Work out the finished part from the listing and answer in its coordinate system (mm). A direction names the side the tool comes from. Round coordinates to 2 decimals unless told otherwise and drop trailing zeros. Order: outer loops, then holes, each group sorted by start corner. A loop starts at its lowest first (then second) coordinate and runs counter-clockwise, first axis right, second up. Notation, with made-up numbers: (25, -33.5) -> (76, -33.5) arc R26 ccw to (76, -7.5) -> close; hole circle Ø2 at (56.25, -8). An arc over 180 degrees is marked (long way). Use a Markdown table: item, result. Add a question column.
Item 1: A cutting plane is placed at C-C, the plane z = 3.4. Determine the outline of the cut face in (x, y), plus the area to 3 significant figures.
Item 2: A cutting plane is placed at B-B, the plane x = 2.5. Determine the outline of the cut face in (y, z), plus the area to 3 significant figures.
Item 3: For a pull along X with two mould halves and no side action, classify faces 4 (the cylindrical face through (-19, -25.44, 1.01)), 5 (the flat face through (30, 1, 0)), 6 (the flat face through (70, -1, 2)) as +X half, -X half, draft (parallel to the pull), parting line (faces both ways), or undercut.
Item 4: A tool of negligible diameter and unlimited length cuts with its end or side. For faces 1 (the flat face through (-70, -1, 2)), 2 (the cylindrical face through (18.94, -25.5, 1.01)), 3 (the flat face through (-27, 1, 2)), from which of +Z, -Z, +X, -X, +Y, -Y can it reach the whole face along a straight path? Write none if from no direction.
Item 5: Find the intervals of material crossed by L1, parallel to Y at x = -34.5, z = 2.9; L2, parallel to X at y = 10, z = 0.9; L3, parallel to X at y = -17, z = 2.35, in increasing order. Write a range as [from, to].
Item 6: A cutting plane is placed at A-A, the plane y = -32. Determine the outline of the cut face in (x, z), plus the area to 3 significant figures.
Item 7: A cutting plane is placed at D-D, the plane x = -27.5. Determine the outline of the cut face in (y, z).
from build123d import *

# Parameters (mm, degrees)
SKETCH_1_W          = 140
SKETCH_1_H          = 160
EXTRUDE_1_DEPTH     = 2
SKETCH_2_W          = 140
SKETCH_2_H          = 160
SKETCH_2_W_2        = 80
SKETCH_2_H_2        = 100
EXTRUDE_2_DEPTH     = 2
CUT_EXTRUDE_1_DEPTH = 2


with BuildPart() as part:
    # 草图1 → 凸台-拉伸1 (new body)
    with BuildSketch(Plane.XY):
        Rectangle(SKETCH_1_W, SKETCH_1_H)
    extrude(amount=EXTRUDE_1_DEPTH)

    # 草图2 → 凸台-拉伸2 (add)
    with BuildSketch(Plane.XY.offset(2)):
        Rectangle(SKETCH_2_W, SKETCH_2_H)
        Rectangle(SKETCH_2_W_2, SKETCH_2_H_2, mode=Mode.SUBTRACT)
    extrude(amount=EXTRUDE_2_DEPTH)

    # 草图4 → 切除-拉伸1 (cut)
    with BuildSketch(Plane.XY.offset(2)):
        with BuildLine():
            Line((-10.8, -34.2), (-6.8, -34.2))
            Line((-6.8, -34.2), (6.8, -34.2))
            Line((6.8, -34.2), (10.8, -34.2))
            Line((10.8, -34.2), (11.2, -34.2))
            Line((11.2, -34.2), (15.2, -34.2))
            Line((15.2, -34.2), (15.2, -26.7))
            Line((15.2, -26.7), (16, -26.7))
            ThreePointArc((16, -26.7), (18.969848481, -25.469848481), (20.2, -22.5))
            Line((20.2, -22.5), (20.2, 29.5))
            ThreePointArc((20.2, 29.5), (18.969848481, 32.469848481), (16, 33.7))
            Line((16, 33.7), (-16, 33.7))
            ThreePointArc((-16, 33.7), (-18.969848481, 32.469848481), (-20.2, 29.5))
            Line((-20.2, 29.5), (-20.2, -22.5))
            ThreePointArc((-20.2, -22.5), (-18.969848481, -25.469848481), (-16, -26.7))
            Line((-16, -26.7), (-15.2, -26.7))
            Line((-15.2, -26.7), (-15.2, -34.2))
            Line((-15.2, -34.2), (-11.2, -34.2))
            Line((-11.2, -34.2), (-10.8, -34.2))
        make_face()
    extrude(amount=-CUT_EXTRUDE_1_DEPTH, mode=Mode.SUBTRACT)


solid = part.part
Reported:
| question | item | result |
|---|---|---|
| 1 | outline | (-70, -80) -> (70, -80) -> (70, 80) -> (-70, 80) -> close; hole (-40, -50) -> (40, -50) -> (40, 50) -> (-40, 50) -> close |
| 1 | area | 14,400 mm² |
| 2 | outline | (-80, 0) -> (-34.2, 0) -> (-34.2, 2) -> (-50, 2) -> (-50, 4) -> (-80, 4) -> close; (33.7, 0) -> (80, 0) -> (80, 4) -> (50, 4) -> (50, 2) -> (33.7, 2) -> close |
| 2 | area | 304 mm² |
| 3 | face 4 | undercut |
| 3 | face 5 | draft |
| 3 | face 6 | +X half |
| 4 | face 1 | +Z, -Z, -X, +Y, -Y |
| 4 | face 2 | +Z, -Z |
| 4 | face 3 | +Z |
| 5 | L1 | [-80, -50], [50, 80] |
| 5 | L2 | [-70, -20.2], [20.2, 70] |
| 5 | L3 | [-70, -40], [40, 70] |
| 6 | outline | (-70, 0) -> (-15.2, 0) -> (-15.2, 2) -> (-40, 2) -> (-40, 4) -> (-70, 4) -> close; (15.2, 0) -> (70, 0) -> (70, 4) -> (40, 4) -> (40, 2) -> (15.2, 2) -> close |
| 6 | area | 339 mm² |
| 7 | outline | (-80, 0) -> (80, 0) -> (80, 4) -> (50, 4) -> (50, 2) -> (-50, 2) -> (-50, 4) -> (-80, 4) -> close |
